```python
from build123d import *

# Parameters (mm, degrees)
F0_R     = 25
F1_DEPTH = 500
F2_R     = 5
F3_DEPTH = 5
F4_R     = 5
F5_DEPTH = 5
F6_R     = 5
F7_R     = 5


with BuildPart() as f1:
    # F0 (on Front) → F1 (new body)
    with BuildSketch(Plane.XZ):
        with Locations((41.250005, 34.250002)):
            Circle(F0_R)
    extrude(amount=F1_DEPTH)

    # F2 (on face) → F3 (join)
    with BuildSketch(Plane(origin=(0, 0, 0), x_dir=(-1, 0, 0), z_dir=(0, 1, 0))):
        with Locations((-41.250005, 34.250002)):
            Circle(F2_R)
    extrude(amount=F3_DEPTH)

    # F4 (on face) → F5 (join)
    with BuildSketch(Plane.XZ.offset(500)):
        with Locations((41.250005, 34.250002)):
            Circle(F4_R)
    extrude(amount=F5_DEPTH)

    # F6
    f6_edges = [f1.edges().sort_by_distance(p)[0] for p in [
        (16.250005, 0, 34.250002),
    ]]
    fillet(f6_edges, radius=F6_R)

    # F7
    f7_edges = [f1.edges().sort_by_distance(p)[0] for p in [
        (16.250005, -500, 34.250002),
    ]]
    fillet(f7_edges, radius=F7_R)


solid = f1.part
```
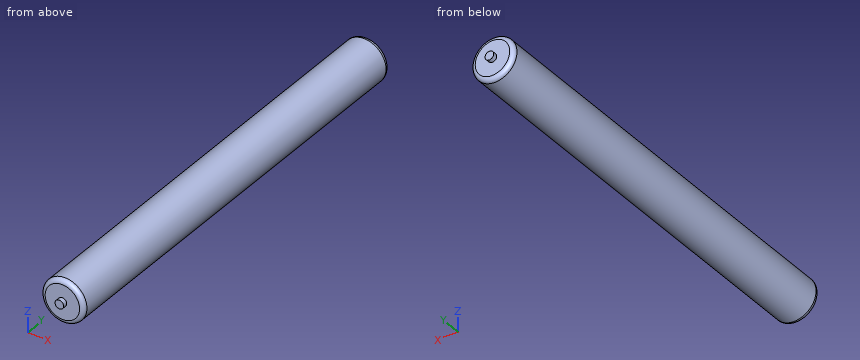
Source: CAD feature listing. Evaluate the final solid. Frame: model axes, mm. Coordinates: 2 decimals unless noted, no trailing zeros. Write each loop counter-clockwise with the first axis right and the second up, starting at its lowest first coordinate (ties: lowest second). Pieces come first, ordered by that corner, then holes. Notation, with made-up numbers: (-12, -20.75) -> (26, -20.75) arc R25 cw to (26, 0.25) -> close; hole circle Ø3 at (51.5, 35.25). An arc over 180 degrees is marked (long way). Return JSON: item names as keys, results as strings. Group by question number.
1) Section query A-A, the plane y = -474. Return loops of the section in (x, z), plus the area to 3 significant figures.
2) Ray query, line 1 along Y through (x, z) = (41, 22); line 2 along X through (y, z) = (-293.5, 34.5); line 3 along Z through (x, y) = (41.5, -142.5). Return the intervals inside material, ascending.
3) Contact query for flat-ended pins moving along their axis: P1, Ø12, axis at x = 47, z = 53, coming from the +Y side; P2, Ø1.5, axis at x = 24, z = 34.5, coming from the -Y side; P3, Ø2, axis at x = 29.5, y = -285.5, coming from the +Z side; P4, Ø10, axis at x = 38.5, z = 27, coming from the +Y side. Output: stop coordinate, or through.
From the geometry:
{
 "1": {"outline": "circle Ø50 at (41.25, 34.25)", "area": "1,960 mm²"},
 "2": {"line 1": "-500 to 0", "line 2": "16.25 to 66.25", "line 3": "9.25 to 59.25"},
 "3": {"P1": "y = 0", "P2": "y = -500", "P3": "z = 56.82", "P4": "y = 5"}
}
